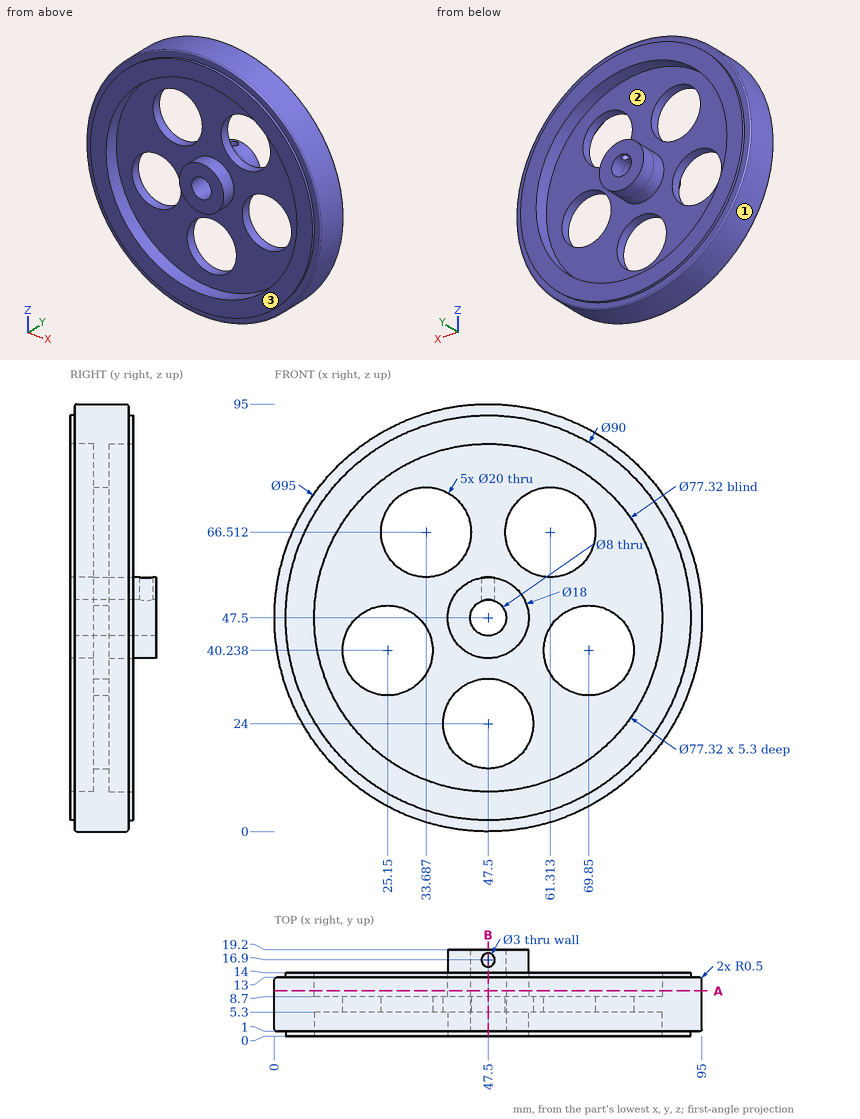
Here's the drawing with two shaded views (mm, measured from the low corner). I have some questions. Coordinates: 2 decimals unless noted, no trailing zeros. Write each loop counter-clockwise with the first axis right and the second up, starting at its lowest first coordinate (ties: lowest second). Pieces come first, ordered by that corner, then holes. Notation, with made-up numbers: (84, 0.5) -> (133, 0.5) arc R12 ccw to (133, 16.5) -> close; hole circle Ø10 at (15, 19). An arc over 180 degrees is marked (long way). One line per question, with ' | ' between items. Start each with the question number.
1. If we section it at A-A (y = 10): Please give me the cut outline in (x, z), and give its area (3 significant figures).
2. If we section it at B-B (x = 47.5): Count the separate pieces of the cut face and the enclosed holes in it, and give its area (3 significant figures).
3. Will these pins go through, and if not, where does the flat tip stop? P1, Ø8, axis at x = 33.5, z = 17.5, coming from the -Y side; P2, Ø4, axis at x = 19.5, y = 3, coming from the -Z side; P3, Ø4, axis at x = 22, y = 5, coming from the +Z side.
4. Please list where these lines run through material, in increasing order: line 1 along Z through (x, y) = (40.5, 10.25); line 2 along X through (y, z) = (7.75, 71); line 3 along Z through (x, y) = (41.5, 2).
5. Thinking about a two-plate mould opening in X: for the marked faces 1, 2 and 3, which applies, pulls with the +X half, pulls with the -X half, needs draft (parallel to the pull), parting line crosses it, or undercut?
Return value:
1) outline: circle Ø95 at (47.5, 47.5); circle Ø18 at (47.5, 47.5); hole circle Ø77.32 at (47.5, 47.5); hole circle Ø8 at (47.5, 47.5) | area: 2,600 mm²
2) separate pieces: 4 | enclosed holes: 0 | area: 548 mm²
3) P1: stops at y = 5.3 | P2: stops at z = 7.75 | P3: stops at z = 88.78
4) line 1: z = 0.52 to 9.48, 41.84 to 53.16, 85.52 to 94.48 | line 2: x = 6.22 to 24.75, 42.62 to 52.38, 70.25 to 88.78 | line 3: z = 0.38 to 9.31, 40.79 to 54.21, 85.69 to 94.62
5) face 1: parting line crosses it | face 2: undercut | face 3: needs draft
